Read the model definition and answer for the solid it produces. Units are mm, in the model's axes. A direction names the side the tool comes from. Give positions to 0.01 mm unless a question says otherwise; leave off trailing zeros. Loops run counter-clockwise (first coordinate to the right, second up) from the corner with the lowest first, then second, coordinate; pieces in that order, holes last. Notation, with made-up numbers: (84, 50.5) - (131, 50.5) arc R20 cw to (131, 65.5) - close; hole circle Ø10 at (83.5, 50). An arc over 180 degrees is marked (long way). Write each question's results on one line, items separated by ' | '. Start each with the question number.
Q1. For faces 4 (the flat face through (-49.53, 0, 91)), 5 (the flat face through (-4.572, 0, 26)), 6 (the flat face through (53, 0, 8.952)), determine the directions among +Z, -Z, +X, -X, +Y, -Y from which every point of the face is accessible in a straight line to the end or side of a thin tool.
Q2. The part is cut by section A-A, the plane x = 6.5. Write down the section's boundary in (y, z).
Q3. The part is cut by section D-D, the plane y = -2. State how many separate pieces and enclosed holes the cut face has, plus the area to 3 significant figures.
Q4. The part is cut by section B-B, the plane z = 106.5. Write down the section's boundary in (x, y), plus the area to 3 significant figures.
Q5. The part is cut by section C-C, the plane x = -45.5. Write down the section's boundary in (y, z).
Q6. Find the intervals of material crossed by line 1 (Z direction, x = 5, y = 2.5); line 2 (X direction, y = -1.5, z = 96.5); line 3 (X direction, y = -1, z = 108), in increasing order. Write a range as from..to.
Q7. Given pin 1 (3 mm diameter, centred on x = 2.5, y = -1.5, fed in from +Z); pin 2 (1.8 mm diameter, centred on y = 1, z = -41, fed in from +X); pin 3 (3 mm diameter, centred on x = 6.5, y = 1.5, fed in from -Z), each flat-ended and moving along its own axis, determine where each tip first touches the part or whether it passes through.
Q8. Determine the mould class of faces 1 (the flat face through (0, 0, -45.72)), 2 (the flat face through (4.572, 0, 84)), 3 (the cylindrical face through (-26.255, 0.043, 75.232)) for opening direction Z: +Z half, -Z half, draft (parallel to the pull), parting line (faces both ways), or undercut.
```python
from build123d import *

# Parameters (mm, degrees)
SKETCH1_W           = 6.096
SKETCH1_H           = 7.62
BOSS_EXTRUDE1_DEPTH = 3.048


with BuildPart() as part:
    # Sketch1 → Boss-Extrude1 (new, symmetric)
    with BuildSketch(Plane(origin=(0, 0, 0), x_dir=(1, 0, 0), z_dir=(0, 1, 0))):
        with BuildLine():
            Line((-49.53, 45.72), (-10.668, 45.72))
            Line((-10.668, 45.72), (-10.668, 38.1))
            Line((-10.668, 38.1), (-4.572, 38.1))
            Line((-4.572, 38.1), (-4.572, 45.72))
            Line((-4.572, 45.72), (4.572, 45.72))
            Line((4.572, 45.72), (4.572, 38.1))
            Line((4.572, 38.1), (10.668, 38.1))
            Line((10.668, 38.1), (10.668, 45.72))
            Line((10.668, 45.72), (49.53, 45.72))
            Line((49.53, 45.72), (49.53, 38.1))
            Line((49.53, 38.1), (55.626, 38.1))
            Line((55.626, 38.1), (55.626, -8.951856626))
            Line((55.626, -8.951856626), (49.53, -8.951856626))
            Line((49.53, -8.951856626), (49.53, -16.571856626))
            Line((49.53, -16.571856626), (55.626, -16.571856626))
            Line((55.626, -16.571856626), (55.626, -29.271856626))
            Line((55.626, -29.271856626), (21.019827136, -42.136821893))
            ThreePointArc((21.019827136, -42.136821893), (17.95098831, -44.911778638), (17.631953735, -49.036869377))
            Line((17.631953735, -49.036869377), (25.187729856, -73.287029113))
            ThreePointArc((25.187729856, -73.287029113), (26.234780075, -75.207903536), (27.939063878, -76.579577488))
            ThreePointArc((27.939063878, -76.579577488), (41.468907088, -82.632484358), (55.626, -87.022365809))
            Line((55.626, -87.022365809), (55.626, -132.617292876))
            Line((55.626, -132.617292876), (10.668, -132.617292876))
            Line((10.668, -132.617292876), (10.668, -122.457292876))
            Line((10.668, -122.457292876), (4.572, -122.457292876))
            Line((4.572, -122.457292876), (4.572, -94.642365809))
            Line((4.572, -94.642365809), (10.668, -94.642365809))
            Line((10.668, -94.642365809), (10.668, -87.022365809))
            Line((10.668, -87.022365809), (4.572, -87.022365809))
            Line((4.572, -87.022365809), (4.572, -80.672365809))
            Line((4.572, -80.672365809), (-4.572, -80.672365809))
            Line((-4.572, -80.672365809), (-4.572, -87.022365809))
            Line((-4.572, -87.022365809), (-10.668, -87.022365809))
            Line((-10.668, -87.022365809), (-10.668, -94.642365809))
            Line((-10.668, -94.642365809), (-4.572, -94.642365809))
            Line((-4.572, -94.642365809), (-4.572, -122.457292876))
            Line((-4.572, -122.457292876), (-10.668, -122.457292876))
            Line((-10.668, -122.457292876), (-10.668, -132.617292876))
            Line((-10.668, -132.617292876), (-49.53, -132.617292876))
            Line((-49.53, -132.617292876), (-49.53, -124.997292876))
            Line((-49.53, -124.997292876), (-55.626, -124.997292876))
            Line((-55.626, -124.997292876), (-55.626, -97.057292876))
            Line((-55.626, -97.057292876), (-49.53, -97.057292876))
            Line((-49.53, -97.057292876), (-49.53, -85.359826344))
            ThreePointArc((-49.53, -85.359826344), (-38.527111219, -81.479756652), (-27.939063878, -76.579577488))
            ThreePointArc((-27.939063878, -76.579577488), (-26.234780075, -75.207903536), (-25.187729856, -73.287029113))
            Line((-25.187729856, -73.287029113), (-17.631953735, -49.036869377))
            ThreePointArc((-17.631953735, -49.036869377), (-17.95098831, -44.911778638), (-21.019827136, -42.136821893))
            Line((-21.019827136, -42.136821893), (-55.626, -29.271856626))
            Line((-55.626, -29.271856626), (-55.626, -16.571856626))
            Line((-55.626, -16.571856626), (-49.53, -16.571856626))
            Line((-49.53, -16.571856626), (-49.53, -8.951856626))
            Line((-49.53, -8.951856626), (-55.626, -8.951856626))
            Line((-55.626, -8.951856626), (-55.626, 38.1))
            Line((-55.626, 38.1), (-49.53, 38.1))
            Line((-49.53, 38.1), (-49.53, 45.72))
        make_face()
        with Locations((7.62, -25.461856626)):
            Rectangle(SKETCH1_W, SKETCH1_H, mode=Mode.SUBTRACT)
        with Locations((-7.62, -25.461856626)):
            Rectangle(SKETCH1_W, SKETCH1_H, mode=Mode.SUBTRACT)
    extrude(amount=BOSS_EXTRUDE1_DEPTH, both=True)


solid = part.part
```
Check sheet entries:
1) face 4: -X, +Y, -Y | face 5: +Y, -Y | face 6: +X, +Y, -Y
2) outline: (-3.05, -38.1) - (3.05, -38.1) - (3.05, 21.65) - (-3.05, 21.65) - close; (-3.05, 29.27) - (3.05, 29.27) - (3.05, 87.02) - (-3.05, 87.02) - close; (-3.05, 94.64) - (3.05, 94.64) - (3.05, 122.46) - (-3.05, 122.46) - close
3) separate pieces: 1 | enclosed holes: 2 | area: 15,500 mm^2
4) outline: (-55.63, -3.05) - (-4.57, -3.05) - (-4.57, 3.05) - (-55.63, 3.05) - close; (4.57, -3.05) - (55.63, -3.05) - (55.63, 3.05) - (4.57, 3.05) - close | area: 622 mm^2
5) outline: (-3.05, -45.72) - (3.05, -45.72) - (3.05, 33.04) - (-3.05, 33.04) - close; (-3.05, 84.07) - (3.05, 84.07) - (3.05, 132.62) - (-3.05, 132.62) - close
6) line 1: z = -38.1..21.65, 29.27..87.02, 94.64..122.46 | line 2: x = -49.53..-4.57, 4.57..55.63 | line 3: x = -55.63..-4.57, 4.57..55.63
7) pin 1: stops at z = 80.67 | pin 2: stops at x = 49.53 | pin 3: stops at z = -38.1
8) face 1: -Z half | face 2: draft | face 3: undercut
